from build123d import *

# Parameters (mm, degrees)
SKETCH1_R           = 5
SKETCH1_R_2         = 11
SKETCH1_R_3         = 2
SKETCH1_R_4         = 1.984633097
SKETCH1_R_5         = 1.894356903
SKETCH1_R_6         = 1.6
BOSS_EXTRUDE1_DEPTH = 8


with BuildPart() as part:
    # Sketch1 → Boss-Extrude1 (new body)
    with BuildSketch(Plane.XY):
        with BuildLine():
            Line((-22, -22), (22, -22))
            ThreePointArc((22, -22), (25.535533906, -20.535533906), (27, -17))
            Line((27, -17), (27, 25))
            Line((27, 25), (-27, 25))
            Line((-27, 25), (-27, -17))
            ThreePointArc((-27, -17), (-25.535533906, -20.535533906), (-22, -22))
        make_face()
        with Locations((-19, 0)):
            Circle(SKETCH1_R, mode=Mode.SUBTRACT)
        with Locations((19, 0)):
            Circle(SKETCH1_R, mode=Mode.SUBTRACT)
        Circle(SKETCH1_R_2, mode=Mode.SUBTRACT)
        with Locations((0, 21)):
            Circle(SKETCH1_R_3, mode=Mode.SUBTRACT)
        with Locations((-19, 21)):
            Circle(SKETCH1_R_4, mode=Mode.SUBTRACT)
        with Locations((19, 21)):
            Circle(SKETCH1_R_5, mode=Mode.SUBTRACT)
        with Locations((-15.5, 15.5)):
            Circle(SKETCH1_R_6, mode=Mode.SUBTRACT)
        with Locations((15.5, 15.5)):
            Circle(SKETCH1_R_6, mode=Mode.SUBTRACT)
        with Locations((15.5, -15.5)):
            Circle(SKETCH1_R_6, mode=Mode.SUBTRACT)
        with Locations((-15.5, -15.5)):
            Circle(SKETCH1_R_6, mode=Mode.SUBTRACT)
    extrude(amount=BOSS_EXTRUDE1_DEPTH)


solid = part.part
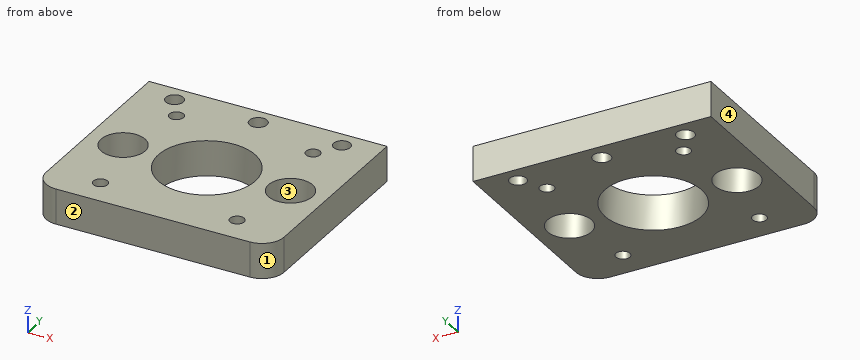
Could you check a few things on this model? Use its own coordinates, in mm. Face numbers are marked on the shaded views. Give positions to 0.01 mm unless a question says otherwise; leave off trailing zeros. Order: outer loops, then holes, each group sorted by start corner. A loop starts at its lowest first (then second) coordinate and runs counter-clockwise, first axis right, second up. Notation, with made-up numbers: (65.25, 49) -> (79.25, 49) arc R23 cw to (79.25, 86) -> close; hole circle Ø1 at (20, -29). An arc over 180 degrees is marked (long way). Answer in a Markdown table with one row per item. Add a question column.
Item 1: Imagine slicing it at A-A (y = 0). List the corners of the cut face in (x, z) for me, and give its area (3 significant figures).
Item 2: Imagine slicing it at B-B (x = -19). List the corners of the cut face in (y, z) for me.
Item 3: We'd pull the mould along X, two halves only. Please class the marked faces 1, 2, 3 and 4: pulls with the +X half, pulls with the -X half, needs draft (parallel to the pull), parting line crosses it, or undercut.
Item 4: Imagine slicing it at D-D (y = 16.5). List the corners of the cut face in (x, z) for me, and give its area (3 significant figures).
Item 5: Imagine slicing it at C-C (z = 6.5). Count the separate pieces of the cut face and the enclosed holes in it, and give its area (3 significant figures).
Item 6: I'm going to push flat-ended pins straight in: P1, Ø2.5, axis at x = 19, y = 21, coming from the +Z side; P2, Ø13, axis at x = 19, y = 0, coming from the +Z side. Where does each tip first touch, or does it pass through?
Item 7: Please list where these lines run through material, in increasing order: probe 1 along Y at (x, z) = (-19, 6); probe 2 along Y at (x, z) = (0, 6.25); probe 3 along X at (y, z) = (-2, 3.75).
Result:
| question | item | result |
|---|---|---|
| 1 | outline | (-27, 0) -> (-24, 0) -> (-24, 8) -> (-27, 8) -> close; (-14, 0) -> (-11, 0) -> (-11, 8) -> (-14, 8) -> close; (11, 0) -> (14, 0) -> (14, 8) -> (11, 8) -> close; (24, 0) -> (27, 0) -> (27, 8) -> (24, 8) -> close |
| 1 | area | 96.0 mm2 |
| 2 | outline | (-22, 0) -> (-5, 0) -> (-5, 8) -> (-22, 8) -> close; (5, 0) -> (19.02, 0) -> (19.02, 8) -> (5, 8) -> close; (22.98, 0) -> (25, 0) -> (25, 8) -> (22.98, 8) -> close |
| 3 | face 1 | pulls with the +X half |
| 3 | face 2 | needs draft |
| 3 | face 3 | undercut |
| 3 | face 4 | pulls with the -X half |
| 4 | outline | (-27, 0) -> (-16.75, 0) -> (-16.75, 8) -> (-27, 8) -> close; (-14.25, 0) -> (14.25, 0) -> (14.25, 8) -> (-14.25, 8) -> close; (16.75, 0) -> (27, 0) -> (27, 8) -> (16.75, 8) -> close |
| 4 | area | 392 mm2 |
| 5 | separate pieces | 1 |
| 5 | enclosed holes | 10 |
| 5 | area | 1,920 mm2 |
| 6 | P1 | through |
| 6 | P2 | z = 8 |
| 7 | probe 1 | -22 to -5, 5 to 19.02, 22.98 to 25 |
| 7 | probe 2 | -22 to -11, 11 to 19, 23 to 25 |
| 7 | probe 3 | -27 to -23.58, -14.42 to -10.82, 10.82 to 14.42, 23.58 to 27 |
